```python
from build123d import *

# Parameters (mm, degrees)
BOSS_EXTRUDE1_DEPTH = 30
FILLET1_R           = 10
FILLET3_RADIUS      = 3.55
FILLET3_LENGTH      = 30


with BuildPart() as part:
    # Sketch1 → Boss-Extrude1 (new body)
    with BuildSketch(Plane.XY):
        with BuildLine():
            Line((5, 0), (5, 8))
            Line((5, 8), (12.1, 8))
            Line((12.1, 8), (12.1, 0))
            ThreePointArc((12.1, 0), (0, -12.1), (-12.1, 0))
            Line((-12.1, 0), (-12.1, 26))
            Line((-12.1, 26), (-5, 26))
            Line((-5, 26), (-5, 0))
            ThreePointArc((-5, 0), (0, -5), (5, 0))
        make_face()
    extrude(amount=-BOSS_EXTRUDE1_DEPTH)

    # Fillet1
    # the kernel refuses this fillet: 10 mm, written as the material it takes off along each edge
    with BuildSketch(Plane(origin=(-12.1, 26, 23.925666135), x_dir=(0, -1, 0), z_dir=(0, 0, -1))) as fillet1_piece_1:
        with BuildLine():
            CenterArc((9.570266454, -10), FILLET1_R, 90, 73.142043978)
            Line((0, -7.1), (-0.191405329, -7.042))
            ThreePointArc((-0.191405329, -7.042), (-0.2, -3.55), (-0.2, 0))
            Line((-0.2, 0), (0, 0.2))
            Line((0, 0.2), (9.570266454, 0.2))
            Line((9.570266454, 0.2), (9.570266454, 0))
        make_face()
    extrude(amount=77.85133227, mode=Mode.SUBTRACT)

    # Fillet3: full round fillet: the end face becomes a half cylinder, R = half its width
    fillet3_face = Plane((8.55, 8, -15), x_dir=(0, 0, 1), z_dir=(0, 1, 0))  # on the end face: x along it, z out of the body
    fillet3_slab = fillet3_face.offset(-FILLET3_RADIUS / 2) * Box(FILLET3_LENGTH, 2 * FILLET3_RADIUS, FILLET3_RADIUS, mode=Mode.PRIVATE)  # the body's end, R deep
    fillet3_round = Plane((8.55, 4.45, -15), x_dir=(0, 1, 0), z_dir=(0, 0, 1)) * Cylinder(FILLET3_RADIUS, FILLET3_LENGTH, mode=Mode.PRIVATE)  # its axis R under the face
    add(fillet3_slab - fillet3_round, mode=Mode.SUBTRACT)


solid = part.part
```
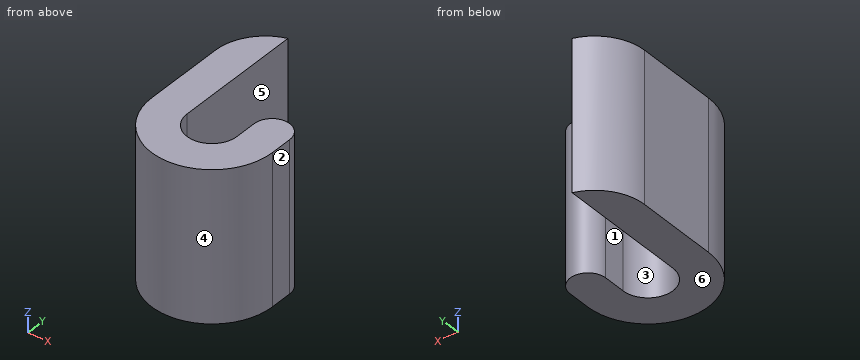
CAD build for the part. Positions are in the model's coordinates, mm. Face numbers are marked on the shaded views. A direction names the side the tool comes from. Round coordinates to 2 decimals unless told otherwise and drop trailing zeros. Write each loop counter-clockwise with the first axis right and the second up, starting at its lowest first coordinate (ties: lowest second). Pieces come first, ordered by that corner, then holes.
Item 1: Mould opens along X. For the marked faces 3, 4, 5 and 6 say: released by +X, released by -X, zero draft, split by the parting line, or undercut.
Filled in:
face 3: undercut
face 4: split by the parting line
face 5: undercut
face 6: zero draft
Item 2: Tool access for the marked faces 1 and 2: list every direction of +Z, -Z, +X, -X, +Y, -Y with a clear straight run to the whole face (end or side of a thin tool).
Filled in:
face 1: +Z, -Z, +Y
face 2: +Z, -Z, +X, +Y, -Y
Item 3: Band-saw the part on B-B on z = -24. Write the cut outline in (x, y).
Filled in:
outline: (-12.1, 0) arc R12.1 ccw to (12.1, 0) - (12.1, 4.45) arc R3.55 ccw to (5, 4.45) - (5, 0) arc R5 cw to (-5, 0) - (-5, 26) arc R10 ccw to (-12.1, 16.43) - close
Item 4: Drop flat-ended pins along their axis: pin 1 Ø8 at (y, z) = (9.5, -10.5) entering from +X; pin 2 Ø6 at (x, z) = (2.5, -11) entering from +Y; pin 3 Ø1 at (y, z) = (15.5, -25) entering from +X. Give the stop position or say it passes through.
Filled in:
pin 1: stops at x = 11.94
pin 2: stops at y = 6.27
pin 3: stops at x = -5
Item 5: Drill centre lines: L1, parallel to X at y = 3, z = -7.25; L2, parallel to X at y = 13, z = -21.25; L3, parallel to X at y = -3, z = -16.25. Where is each one in solid material? Low to high.
Filled in:
L1: x = -12.1 to -5, 5 to 12.1
L2: x = -12.1 to -5
L3: x = -11.72 to -4, 4 to 11.72
Item 6: Band-saw the part on A-A on y = 2.5. Write the cut outline in (x, z), then the cut area to 3 significant figures.
Filled in:
outline: (-12.1, -30) - (-5, -30) - (-5, 0) - (-12.1, 0) - close; (5, -30) - (12.1, -30) - (12.1, 0) - (5, 0) - close
area: 426 mm2
Item 7: Band-saw the part on C-C on x = 0. Write the cut outline in (y, z), then the cut area to 3 significant figures.
Filled in:
outline: (-12.1, -30) - (-5, -30) - (-5, 0) - (-12.1, 0) - close
area: 213 mm2
